For this review, use the dimensioned drawing (mm, ordinates from the lowest corner) and the shaded views. Give positions to 0.01 mm unless a question says otherwise; leave off trailing zeros. Order: outer loops, then holes, each group sorted by start corner. A loop starts at its lowest first (then second) coordinate and runs counter-clockwise, first axis right, second up.
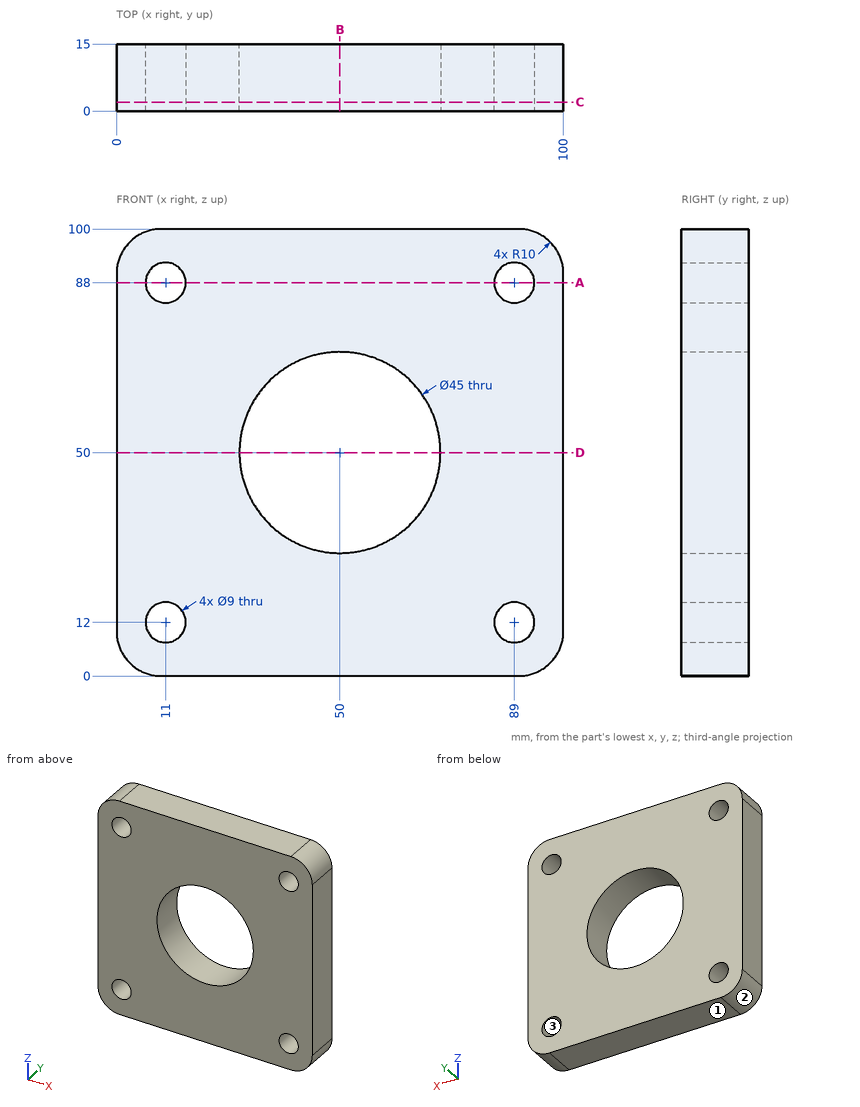
1. Take a section at C-C (y = 2). State the section outline as (x, z) points.
Recorded:
outline: (0, 10) arc R10 ccw to (10, 0) - (90, 0) arc R10 ccw to (100, 10) - (100, 90) arc R10 ccw to (90, 100) - (10, 100) arc R10 ccw to (0, 90) - close; hole circle Ø9 at (11, 12); hole circle Ø9 at (11, 88); hole circle Ø45 at (50, 50); hole circle Ø9 at (89, 12); hole circle Ø9 at (89, 88)
2. Draft analysis for pull direction X (two halves, no side actions). For the marked faces 1, 2 and 3, state which applies: pulls with the +X half, pulls with the -X half, needs draft (parallel to the pull), parting line crosses it, or undercut.
Recorded:
face 1: needs draft
face 2: pulls with the -X half
face 3: undercut
3. Take a section at D-D (z = 50). State the section outline as (x, y) points.
Recorded:
outline: (0, 0) - (27.5, 0) - (27.5, 15) - (0, 15) - close; (72.5, 0) - (100, 0) - (100, 15) - (72.5, 15) - close
4. Take a section at B-B (x = 50). State the section outline as (y, z) points.
Recorded:
outline: (0, 0) - (15, 0) - (15, 27.5) - (0, 27.5) - close; (0, 72.5) - (15, 72.5) - (15, 100) - (0, 100) - close
5. Take a section at A-A (z = 88). State the section outline as (x, y) points, then the cut area to 3 significant figures.
Recorded:
outline: (0, 0) - (6.5, 0) - (6.5, 15) - (0, 15) - close; (15.5, 0) - (84.5, 0) - (84.5, 15) - (15.5, 15) - close; (93.5, 0) - (100, 0) - (100, 15) - (93.5, 15) - close
area: 1,230 mm2
6. For line 1 along Z through (x, y) = (11, 10.5); line 2 along Z through (x, y) = (91, 8); line 3 along Z through (x, y) = (49.5, 11), list the stretches that pass through material, from the lowest coordinate up.
Recorded:
line 1: z = 0 to 7.5, 16.5 to 83.5, 92.5 to 100
line 2: z = 0.05 to 7.97, 16.03 to 83.97, 92.03 to 99.95
line 3: z = 0 to 27.51, 72.49 to 100
